Part model, mm, in its own coordinate system. A direction names the side the tool comes from. Give positions to 0.01 mm unless a question says otherwise; leave off trailing zeros. Order: outer loops, then holes, each group sorted by start corner. A loop starts at its lowest first (then second) coordinate and runs counter-clockwise, first axis right, second up. Notation, with made-up numbers: (-10, -34) - (28, -34) arc R13 cw to (28, -27) - close; hole circle Ø5 at (65, 86). An arc over 180 degrees is marked (long way). One line per item, written item: value.
```python
from build123d import *

# Parameters (mm, degrees)
ESQUISSE1_R             = 2.5
BOSS_EXTRU_1_DEPTH      = 20
ESQUISSE2_W             = 10
ESQUISSE2_H             = 20
ENL_V_MAT_EXTRU_1_DEPTH = 10


with BuildPart() as part:
    # Esquisse1 → Boss.-Extru.1 (new body)
    with BuildSketch(Plane.XY):
        Polygon((-105, 0), (-5, -10), (5, -10), (5, 10), (-5, 10), (-95, 10), (-95, 20), (-105, 20), (-105, 10), align=None)
        with Locations((0, 5)):
            Circle(ESQUISSE1_R, mode=Mode.SUBTRACT)
        with Locations((0, -5)):
            Circle(ESQUISSE1_R, mode=Mode.SUBTRACT)
    extrude(amount=BOSS_EXTRU_1_DEPTH)

    # Esquisse2 → Enlèv. mat.-Extru.1 (cut)
    with BuildSketch(Plane.XY.offset(20)):
        Rectangle(ESQUISSE2_W, ESQUISSE2_H)
    extrude(amount=-ENL_V_MAT_EXTRU_1_DEPTH, mode=Mode.SUBTRACT)


solid = part.part
```
1) Which spindle directions (+Z, -Z, +X, -X, +Y, -Y) get a long thin tool onto all of the face, cutting with end or side? Do faces 5 (the flat face through (0, -10, 5)), 6 (the flat face through (-5, 0, 15)), 7 (the flat face through (-44, 10, 10)). Say none if no direction does.
Outcome:
face 5: +Z, -Z, +X, -X, -Y
face 6: +Z, +X, +Y, -Y
face 7: +Z, -Z, +X, +Y
2) Cut at B-B, the plane z = 5.5. Give the cut face in (x, y).
Outcome:
outline: (-105, 0) - (-5, -10) - (5, -10) - (5, 10) - (-95, 10) - (-95, 20) - (-105, 20) - close; hole circle Ø5 at (0, -5); hole circle Ø5 at (0, 5)
3) Cut at A-A, the plane y = 5. Give the cut face in (x, z), then the cut area to 3 significant figures.
Outcome:
outline: (-105, 0) - (-2.5, 0) - (-2.5, 10) - (-5, 10) - (-5, 20) - (-105, 20) - close; (2.5, 0) - (5, 0) - (5, 10) - (2.5, 10) - close
area: 2,050 mm^2
4) Cut at D-D, the plane y = -3.75. Give the cut face in (x, z), then the cut area to 3 significant figures.
Outcome:
outline: (-67.5, 0) - (-2.17, 0) - (-2.17, 10) - (-5, 10) - (-5, 20) - (-67.5, 20) - close; (2.17, 0) - (5, 0) - (5, 10) - (2.17, 10) - close
area: 1,310 mm^2
5) Mould opens along X. For faces 1 (the flat face through (-51, 2, 0)), 2 (the cylindrical face through (-0.33, 7.48, 4.93)), 3 (the cylindrical face through (-0.33, -2.52, 4.93)), 4 (the flat face through (-95, 15, 10)) say: released by +X, released by -X, zero draft, split by the parting line, or undercut.
Outcome:
face 1: zero draft
face 2: undercut
face 3: undercut
face 4: released by +X
6) Cut at C-C, the plane x = -10. Give the cut face in (y, z), then the cut area to 3 significant figures.
Outcome:
outline: (-9.5, 0) - (10, 0) - (10, 20) - (-9.5, 20) - close
area: 390 mm^2
7) Drill centre lines: line 1 along Y through (x, z) = (0, 6); line 2 along X through (y, z) = (5, 5); line 3 along X through (y, z) = (7, 10.5). Where is each one in solid material? Low to high. Write a range as from..to.
Outcome:
line 1: y = -10..-7.5, -2.5..2.5, 7.5..10
line 2: x = -105..-2.5, 2.5..5
line 3: x = -105..-5
8) Pin check, flat tips, straight feed: pin 1 (8 mm diameter, centred on y = -2, z = 15.5, fed in from +X); pin 2 (1 mm diameter, centred on x = -55.5, z = 18, fed in from +Y); pin 3 (5 mm diameter, centred on x = -73, z = 12.5, fed in from -Y). Stop position of each tip, or through.
Outcome:
pin 1: stops at x = -5
pin 2: stops at y = 10
pin 3: stops at y = -3.45
